Geometry check sheet. Reference: drawing and pictorial views, mm from the part's lowest x, y, z. Round coordinates to 2 decimals unless told otherwise and drop trailing zeros. Order: outer loops, then holes, each group sorted by start corner. A loop starts at its lowest first (then second) coordinate and runs counter-clockwise, first axis right, second up.
(1) Sectioned sample at C-C (x = 10.75). Record the boundary of the cut face in (y, z) (1 decimal).
(2) Sectioned sample at A-A (x = 2.25). Record the boundary of the cut face in (y, z), plus the area to 3 significant figures.
(3) Sectioned sample at B-B (y = 1.5). Record the boundary of the cut face in (x, z).
(4) Material ranges on line 1 along Z through (x, y) = (4.5, 7); line 2 along Y through (x, z) = (3.5, 0.1) (1 decimal); line 3 along Y through (x, z) = (2, 0.3), recorded low to high.
(5) Go/stop test with flat-tipped pins: pin 1 (2.5 mm diameter, centred on x = 19.168, y = 2.168, fed in from -Z); pin 2 (0.8 mm diameter, centred on x = 11.5, z = 2, fed in from -Y); pin 3 (0.8 mm diameter, centred on x = 10, z = 2, fed in from +Y); pin 4 (0.5 mm diameter, centred on y = 7.5, z = 1.5, fed in from -X). Record where each tip stops, or that it passes through.
(6) Sectioned sample at D-D (y = 6.75). Record the boundary of the cut face in (x, z).
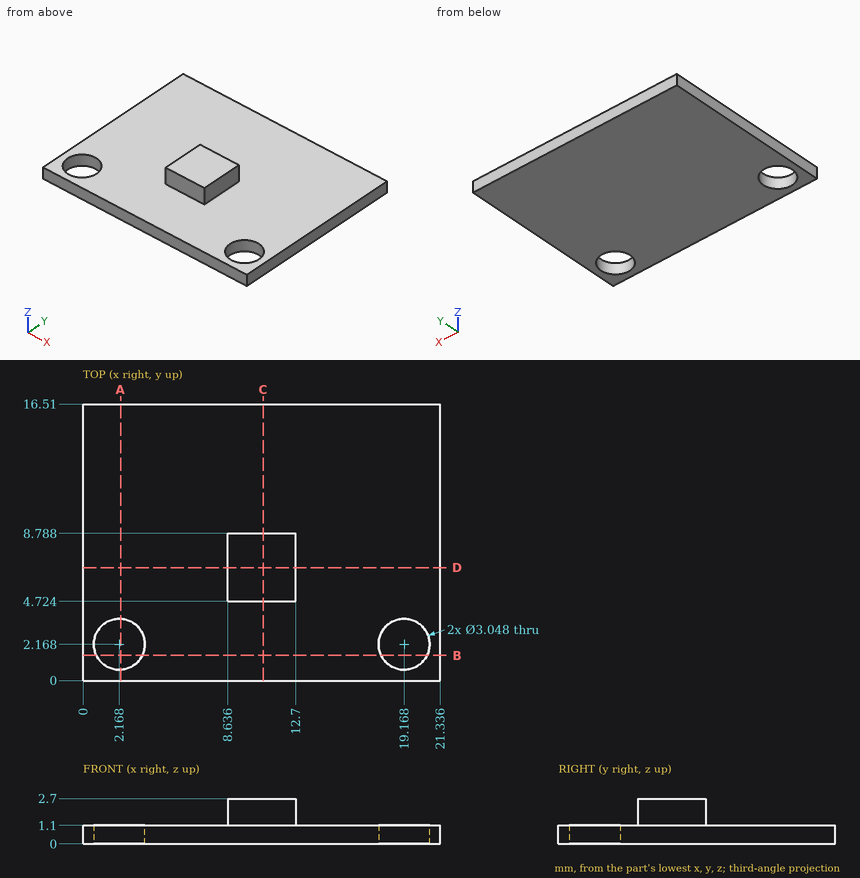
Answer below:
1. outline: (0, 0) - (16.5, 0) - (16.5, 1.1) - (8.8, 1.1) - (8.8, 2.7) - (4.7, 2.7) - (4.7, 1.1) - (0, 1.1) - close
2. outline: (0, 0) - (0.65, 0) - (0.65, 1.1) - (0, 1.1) - close; (3.69, 0) - (16.51, 0) - (16.51, 1.1) - (3.69, 1.1) - close
2. area: 14.8 mm2
3. outline: (0, 0) - (0.8, 0) - (0.8, 1.1) - (0, 1.1) - close; (3.54, 0) - (17.8, 0) - (17.8, 1.1) - (3.54, 1.1) - close; (20.54, 0) - (21.34, 0) - (21.34, 1.1) - (20.54, 1.1) - close
4. line 1: z = 0 to 1.1
4. line 2: y = 0 to 1.4, 2.9 to 16.5
4. line 3: y = 0 to 0.65, 3.68 to 16.51
5. pin 1: passes through
5. pin 2: stops at y = 4.72
5. pin 3: stops at y = 8.79
5. pin 4: stops at x = 8.64
6. outline: (0, 0) - (21.34, 0) - (21.34, 1.1) - (12.7, 1.1) - (12.7, 2.7) - (8.64, 2.7) - (8.64, 1.1) - (0, 1.1) - close
